The figure shows three views and two pictorial views of one solid part (mm, origin at its lowest corner). Answer the questions. A direction names the side the tool comes from. Coordinates: 2 decimals unless noted, no trailing zeros. Order: outer loops, then holes, each group sorted by start corner. A loop starts at its lowest first (then second) coordinate and runs counter-clockwise, first axis right, second up. Notation, with made-up numbers: M 4.25,-13.5 L 38.25,-13.5 A22 ccw 38.25,20.5 Z; hole C -2,-3.5 d8. An arc over 180 degrees is marked long. Answer in a Markdown table with one row per item. Add a question column.
Item 1: Consider line 1 (Y direction, x = 13, z = 9); line 2 (X direction, y = 18.75, z = 5.25); line 3 (Z direction, x = 4.5, y = 13.25). Determine where each line is inside the solid, lowest interval first. Write a range as from..to.
Item 2: The part is cut by section B-B (y = 10). Write down the section's boundary in (x, z), then the cut area to 3 significant figures.
Item 3: The part is cut by section A-A (z = 1.25). Write down the section's boundary in (x, y), then the cut area to 3 significant figures.
Item 4: The part is cut by section D-D (x = 13). Write down the section's boundary in (y, z).
Item 5: Which of the six approach directions +Z, -Z, +X, -X, +Y, -Y give full straight-line access (tool end or side, diameter ignored) to the marked faces 1, 2, 3, 4 and 5?
Item 6: The mould has two halves that part along X. Classify the marked faces 6, 7 and 8: released by +X, released by -X, zero draft, split by the parting line, or undercut.
Item 7: The part is cut by section C-C (z = 9.5). Write down the section's boundary in (x, y), then the cut area to 3 significant figures.
Item 8: Flat-ended cylindrical pins translate along their axes: pin 1 Ø0.9 at (x, z) = (2, 7) entering from +Y; pin 2 Ø5 at (x, y) = (13.5, 10.5) entering from -Z; pin 3 Ø0.9 at (x, z) = (25, 5) entering from -Y. Find the tip coordinate at first contact, or state that the pin passes through.
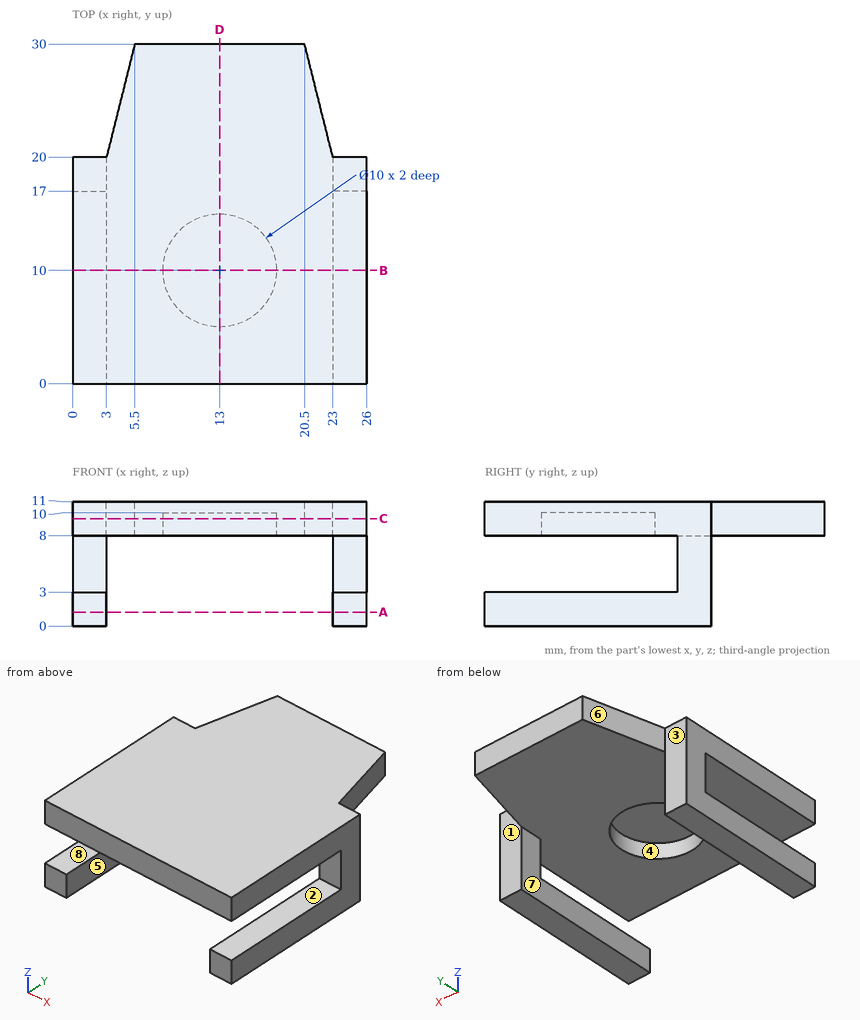
Reply:
| question | item | result |
|---|---|---|
| 1 | line 1 | y = 0..5, 15..30 |
| 1 | line 2 | x = 0..3, 23..26 |
| 1 | line 3 | z = 8..11 |
| 2 | outline | M 0,0 L 3,0 L 3,3 L 0,3 Z; M 0,8 L 8,8 L 8,10 L 18,10 L 18,8 L 26,8 L 26,11 L 0,11 Z; M 23,0 L 26,0 L 26,3 L 23,3 Z |
| 2 | area | 76.0 mm2 |
| 3 | outline | M 0,0 L 3,0 L 3,20 L 0,20 Z; M 23,0 L 26,0 L 26,20 L 23,20 Z |
| 3 | area | 120 mm2 |
| 4 | outline | M 0,8 L 5,8 L 5,10 L 15,10 L 15,8 L 30,8 L 30,11 L 0,11 Z |
| 5 | face 1 | +Z, -Z, +X, +Y |
| 5 | face 2 | +X, -X, -Y |
| 5 | face 3 | +Z, -Z, -X, +Y |
| 5 | face 4 | -Z |
| 5 | face 5 | -Z, +Y, -Y |
| 6 | face 6 | released by -X |
| 6 | face 7 | undercut |
| 6 | face 8 | zero draft |
| 7 | outline | M 0,0 L 26,0 L 26,20 L 23,20 L 20.5,30 L 5.5,30 L 3,20 L 0,20 Z; hole C 13,10 d10 |
| 7 | area | 616 mm2 |
| 8 | pin 1 | stops at y = 20 |
| 8 | pin 2 | stops at z = 10 |
| 8 | pin 3 | stops at y = 17 |
